Autodesk Inventor part; units mm, degrees
ref_plane "YZ Plane" through (0, 0, 0) normal (1, 0, 0) x (0, 1, 0)
ref_plane "XZ Plane" through (0, 0, 0) normal (0, 1, 0) x (-1, 0, 0)
ref_plane "XY Plane" through (0, 0, 0) normal (0, 0, 1) x (1, 0, 0)
sketch "Sketch1" plane through (0, 0, 0) normal (0, 0, 1) x (1, 0, 0)
  line L0 (-6.5, -6.5) -> (6.5, -6.5)
  line L1 (6.5, -6.5) -> (6.5, 6.5)
  line L2 (6.5, 6.5) -> (-6.5, 6.5)
  line L3 (-6.5, 6.5) -> (-6.5, -6.5)
  line L4 (-6.5, -6.5) -> (6.5, 6.5) construction
  line L5 (6.5, -6.5) -> (-6.5, 6.5) construction
  line L6 (-5.75, -5.75) -> (5.75, -5.75)
  line L7 (5.75, -5.75) -> (5.75, 5.75)
  line L8 (5.75, 5.75) -> (-5.75, 5.75)
  line L9 (-5.75, 5.75) -> (-5.75, -5.75)
  point P0 (0, 0)
  dimension "d0" = 13
  dimension "d1" = 13
  dimension "d2" = 0.75
extrude "Extrusion1" add sketch "Sketch1" along normal blind 7.5 contours L9 L8 L7 L6
extrude "Extrusion2" add sketch "Sketch1" along normal blind 7
sketch "Sketch2" plane through (0, 0, 7.5) normal (0, 0, 1) x (1, 0, 0)
  line L0 (5.75, 5.75) -> (-5.75, 5.75)
  line L1 (-5.75, -5.75) -> (5.75, -5.75)
  line L2 (5.75, -5.75) -> (5.75, 5.75)
  line L3 (5.75, 5.75) -> (-5.75, 5.75)
  line L4 (-5.75, 5.75) -> (-5.75, -5.75)
  line L5 (-5.75, -5.75) -> (5.75, 5.75) construction
  line L6 (5.75, -5.75) -> (-5.75, 5.75) construction
  line L7 (-3.75, -3.75) -> (3.75, -3.75)
  line L8 (3.75, -3.75) -> (3.75, 3.75)
  line L9 (3.75, 3.75) -> (-3.75, 3.75)
  line L10 (-3.75, 3.75) -> (-3.75, -3.75)
  line L11 (-4.75, 4.75) -> (4.75, 4.75)
  line L12 (4.75, 4.75) -> (4.75, -4.75)
  line L13 (4.75, -4.75) -> (-4.75, -4.75)
  line L14 (-4.75, -4.75) -> (-4.75, 4.75)
  line L15 (-2.75, 2.75) -> (2.75, 2.75)
  line L16 (2.75, 2.75) -> (2.75, -2.75)
  line L17 (2.75, -2.75) -> (-2.75, -2.75)
  line L18 (-2.75, -2.75) -> (-2.75, 2.75)
  point P0 (0, 0)
  dimension "d7" = 2
  dimension "d10" = 1
  dimension "d14" = 1
extrude "Extrusion3" cut sketch "Sketch2" against normal through all contours L15 L16 L17 L18
sketch "Sketch6" plane through (0, 0, 0) normal (0, 0, -1) x (-1, 0, 0)
  line L0 (2.75, -2.75) -> (2.75, 2.75)
  line L1 (-2.75, -2.75) -> (2.75, -2.75)
  line L2 (2.75, -2.75) -> (2.75, 2.75)
  line L3 (2.75, 2.75) -> (-2.75, 2.75)
  line L4 (-2.75, 2.75) -> (-2.75, -2.75)
  line L5 (-2.75, -2.75) -> (2.75, 2.75) construction
  line L6 (2.75, -2.75) -> (-2.75, 2.75) construction
  line L7 (-3.75, 3.75) -> (3.75, 3.75)
  line L8 (3.75, 3.75) -> (3.75, -3.75)
  line L9 (3.75, -3.75) -> (-3.75, -3.75)
  line L10 (-3.75, -3.75) -> (-3.75, 3.75)
  line L11 (6.5, -6.5) -> (-6.5, -6.5)
  line L12 (-3.75, -3.75) -> (3.75, -3.75)
  line L13 (3.75, -3.75) -> (3.75, -6.5)
  line L14 (3.75, -6.5) -> (-3.75, -6.5)
  line L15 (-3.75, -6.5) -> (-3.75, -3.75)
  line L16 (-1.75, 1.75) -> (1.75, 1.75)
  line L17 (1.75, 1.75) -> (1.75, -1.75)
  line L18 (1.75, -1.75) -> (-1.75, -1.75)
  line L19 (-1.75, -1.75) -> (-1.75, 1.75)
  point P0 (0, 0)
  dimension "d25" = 1
  dimension "d36" = 1
extrude "Extrusion9" add sketch "Sketch6" against normal blind 6 contours L1 L4 L3 L0
sketch "Sketch7" plane through (0, 0, 0) normal (0, 0, -1) x (-1, 0, 0)
  line L0 (6.5, -6.5) -> (-6.5, -6.5)
  line L1 (-3.5, -6.5) -> (3.5, -6.5)
  line L2 (3.5, -6.5) -> (3.5, 2.35)
  line L3 (3.5, 2.35) -> (-3.5, 2.35)
  line L4 (-3.5, 2.35) -> (-3.5, -6.5)
  line L5 (-6.5, -6.5) -> (-6.5, 6.5)
  line L6 (6.5, 6.5) -> (6.5, -6.5)
  line L7 (-1.75, 1.75) -> (1.75, 1.75)
  point P0 (0, 0)
  dimension "d47" = 3
  dimension "d48" = 3
  dimension "d49" = 0.6
extrude "Extrusion10" cut sketch "Sketch7" against normal blind 5
chamfer "Chamfer5" distance 1 angle 45 4 edges at (-1.75, 0, 6) (0, -1.75, 6) (1.75, 0, 6) (0, 1.75, 6)
sketch "Sketch8" plane through (0, 0, 5) normal (0, 0, -1) x (-1, 0, 0)
  point P0 (0, 0)
sketch "Sketch9" plane through (0, 0, 0) normal (0, 0, -1) x (-1, 0, 0)
  line L0 (-6.5, 6.5) -> (6.5, 6.5)
  line L1 (6.5, 6.5) -> (6.5, -6.5)
  line L2 (-6.5, 6.5) -> (6.5, 6.5)
  line L3 (6.5, 6.5) -> (6.5, -6.5)
  line L4 (6.5, -6.5) -> (-6.5, -6.5)
  line L5 (-6.5, -6.5) -> (-6.5, 6.5)
  line L6 (-5.5, 5.5) -> (5.5, 5.5)
  line L7 (5.5, 5.5) -> (5.5, -5.5)
  line L8 (5.5, -5.5) -> (-5.5, -5.5)
  line L9 (-5.5, -5.5) -> (-5.5, 5.5)
  point P0 (0, 0)
  dimension "d50" = 1
extrude "Extrusion11" cut sketch "Sketch9" against normal blind 1
sketch "Sketch10" plane through (-3.5, 2.35, 0) normal (0, -1, 0) x (1, 0, 0)
  line L0 (-2, 0) -> (9, 0)
  line L1 (4.5, 3) -> (2.5, 3)
  line L2 (2.5, 3) -> (2.5, 0)
  line L3 (2.5, 0) -> (4.5, 0)
  line L4 (4.5, 0) -> (4.5, 3)
  point P0 (3.5, 0)
  point P1 (3.5, 0)
  point P2 (4.5, 0)
  dimension "d53" = 3
  dimension "d54" = 2
  dimension "d55" = 1
extrude "Extrusion12" add sketch "Sketch10" along normal blind 4.5
sketch "Sketch11" plane through (-6.5, 6.5, 7) normal (0, 1, 0) x (1, 0, 0)
  line L0 (13, 6) -> (13, 0)
  line L1 (13, 0) -> (15, 0)
  line L2 (15, 0) -> (15, 2)
  line L3 (15, 2) -> (13, 2)
  line L4 (13, 2) -> (13, 0)
  line L5 (0, 6) -> (0, 0)
  line L6 (0, 6) -> (0, 3)
  line L7 (0, 4.5) -> (-2, 4.5)
  line L8 (-2, 4.5) -> (0, 3)
  line L9 (-2, 4.5) -> (0, 6)
  point P0 (6.5, 7)
  point P1 (13, 2)
  dimension "d58" = 2
  dimension "d59" = 2
  dimension "d60" = 2
extrude "Extrusion13" add sketch "Sketch11" against normal blind 13
sketch "Sketch12" plane through (-5.5, 5.5, 0) normal (0, 1, 0) x (1, 0, 0)
  line L0 (0, 0) -> (11, 0)
  line L1 (11, 0) -> (11, -7.4478)
  line L2 (11, -7.4478) -> (0, -7.4478)
  line L3 (0, -7.4478) -> (0, 0)
  line L4 (-0.25, -7.5) -> (11.25, -7.5)
  line L5 (0, 0) -> (11, 0)
  line L6 (11, 0) -> (11, -7.5)
  line L7 (11, -7.5) -> (0, -7.5)
  line L8 (0, -7.5) -> (0, 0)
  point P0 (5.5, 0)
extrude "Extrusion14" add sketch "Sketch12" along normal blind 1
sketch "Sketch13" plane through (0, 0, 7.5) normal (0, 0, 1) x (1, 0, 0)
  line L0 (5.75, 5.75) -> (5.5, 5.75)
  line L1 (-5.5, 6.5) -> (-5.5, -5.5)
  line L2 (5.5, 5.75) -> (-5.5, 5.75)
  line L3 (-5.5, 5.75) -> (-5.5, -5.5)
  line L4 (-5.5, -5.5) -> (5.5, -5.5)
  line L5 (5.5, -5.5) -> (5.5, 5.75)
  line L6 (5.75, -5.75) -> (-5.75, -5.75)
  line L7 (-5.75, -5.75) -> (-5.75, 6)
  line L8 (-5.75, 6) -> (5.75, 6)
  line L9 (5.75, 6) -> (5.75, -5.75)
  point P0 (0, 0)
  point P1 (-5.5, 6)
extrude "Extrusion15" cut sketch "Sketch13" against normal blind 0.5 contours L9 L6 L7 L8 L1 L4 L5 L0
sketch "Sketch14" plane through (0, 0, 7.5) normal (0, 0, 1) x (1, 0, 0)
  line L0 (5.5, 6.5) -> (-5.5, 6.5)
  line L1 (-5.5, 6.5) -> (5.5, 6.5)
  line L2 (5.5, 6.5) -> (5.5, -5.5)
  line L3 (5.5, -5.5) -> (-5.5, -5.5)
  line L4 (-5.5, -5.5) -> (-5.5, 6.5)
  line L5 (-3.25, 3.25) -> (-3.25, -3.25)
  line L6 (-3.25, -3.25) -> (3.25, -3.25)
  line L7 (-3.25, 3.25) -> (3.25, 3.25)
  line L8 (3.25, 3.25) -> (3.25, -3.25)
  line L9 (3.25, -3.25) -> (-3.25, -3.25)
  line L10 (-3.25, -3.25) -> (-3.25, 3.25)
  point P0 (0, 0)
extrude "Extrusion16" add sketch "Sketch14" along normal blind 0.5
sketch "Sketch15" plane through (0, 0, 7) normal (0, 0, 1) x (1, 0, 0)
  line L0 (5.5, 6.5) -> (5.5, -5.5)
  line L1 (5.5, 6.5) -> (-5.5, 6.5)
  line L2 (-5.5, 6.5) -> (-5.5, -5.5)
  line L3 (-5.5, -5.5) -> (5.5, -5.5)
  line L4 (5.5, -5.5) -> (5.5, 6.5)
  line L5 (5.75, -5.75) -> (-5.75, -5.75)
  line L6 (-5.75, -5.75) -> (-5.75, 6.75)
  line L7 (-5.75, 6.75) -> (5.75, 6.75)
  line L8 (5.75, 6.75) -> (5.75, -5.75)
  line L9 (5.75, 6.5) -> (-5.75, 6.5)
  point P0 (0, 0)
  dimension "d69" = 0.25
extrude "Extrusion17" add sketch "Sketch15" along normal blind 1 contours L9 L8 L5 L6 L2 L3 L0
fillet "Fillet1" radius 1 8 edges at (0, 2.75, 7.5) (2.75, 0, 7.5) (-2.75, 0, 7.5) (0, -2.75, 7.5) (0, 3.25, 8) (-3.25, 0, 8) (0, -3.25, 8) (3.25, 0, 8)
properties part number "NV_module" material "PET Plastic"
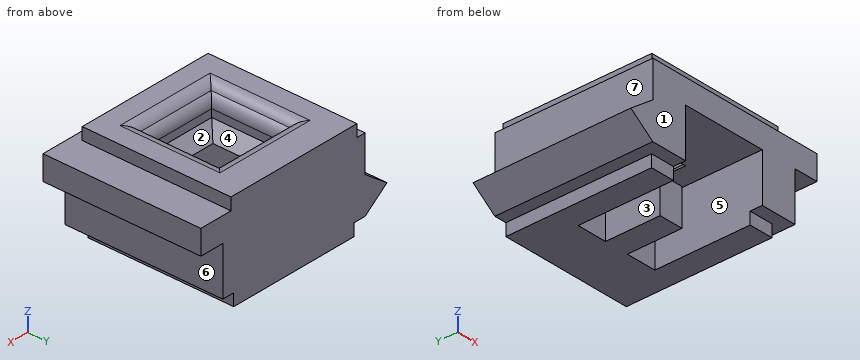
Input: part model. Units: mm. Frame: model coordinates. Face numbers are marked on the shaded views. A direction names the side the tool comes from. Give positions to 0.01 mm unless a question says otherwise; leave off trailing zeros. Loops run counter-clockwise (first coordinate to the right, second up) from the corner with the lowest first, then second, coordinate; pieces in that order, holes last. Notation, with made-up numbers: (56, -4) -> (76, -4) arc R21 cw to (76, 28) -> close; hole circle Ø7 at (-1, 6.25). An arc over 180 degrees is marked (long way). Answer as a JSON object with one key per item and string values. Group by question number.
Item 1: Line query: probe 1 along Y at (x, z) = (0.5, 3.5); probe 2 along Z at (x, y) = (7.25, -4); probe 3 along X at (y, z) = (-4.5, 5.5). Output: solid intervals per line, ascending.
Item 2: Reachability of the marked faces 4, 5, 6 and 7 from +Z, -Z, +X, -X, +Y, -Y: full face, straight path, thin tool, end or side. Return the list, or none.
Item 3: Cut plane C-C, the plane z = 7.75. Return the cut outline in (x, y).
Item 4: Pull-direction query (Y, two-part tool) for the marked faces 1, 2 and 3; classes: released by +Y, released by -Y, zero draft, split by the parting line, or undercut.
Item 5: Cut plane D-D, the plane z = 4.5. Return the cut outline in (x, y), and give its area (3 significant figures).
Item 6: Pin query (flat end, axial travel): P1, Ø1, axis at x = -6.5, y = 4.5, coming from the +Z side; P2, Ø4, axis at x = -1, z = 2, coming from the -Y side; P3, Ø0.6, axis at x = 0.5, y = 0, coming from the +Z side. Return the tip coordinate at first contact, or that it passes through.
Item 7: Cut plane B-B, the plane y = -4.5. Return the cut outline in (x, z), and give its area (3 significant figures).
Checks:
{
 "1": {"probe 1": "y = 2.35 to 6.5", "probe 2": "z = 5 to 7", "probe 3": "x = -6.5 to 8.5"},
 "2": {"face 4": "+Z", "face 5": "-Z, -Y", "face 6": "-Z, +X, +Y, -Y", "face 7": "+Z, -X, +Y, -Y"},
 "3": {"outline": "(-5.75, -5.75) -> (5.75, -5.75) -> (5.75, 6.5) -> (-5.75, 6.5) -> close; hole (-3.45, -3.45) -> (3.45, -3.45) -> (3.45, 3.45) -> (-3.45, 3.45) -> close"},
 "4": {"face 1": "released by -Y", "face 2": "undercut", "face 3": "zero draft"},
 "5": {"outline": "(-6.5, -6.5) -> (-3.5, -6.5) -> (-3.5, 2.35) -> (3.5, 2.35) -> (3.5, -6.5) -> (6.5, -6.5) -> (6.5, 6.5) -> (-6.5, 6.5) -> close", "area": "107 mm²"},
 "6": {"P1": "stops at z = 7", "P2": "stops at y = -2.15", "P3": "stops at z = 3"},
 "7": {"outline": "(-8.5, 2.5) -> (-6.5, 1) -> (-5.5, 1) -> (-5.5, 0) -> (-3.5, 0) -> (-3.5, 5) -> (3.5, 5) -> (3.5, 0) -> (5.5, 0) -> (5.5, 1) -> (6.5, 1) -> (6.5, 5) -> (8.5, 5) -> (8.5, 7) -> (5.75, 7) -> (5.75, 8) -> (-5.75, 8) -> (-5.75, 7) -> (-6.5, 7) -> (-6.5, 4) -> close", "area": "72.5 mm²"}
}
